```python
from build123d import *

# Parameters (mm, degrees)
CROQUIS1_R              = 1
SALIENTE_EXTRUIR1_DEPTH = 10
REDONDEO1_R             = 10


with BuildPart() as part:
    # Croquis1 → Saliente-Extruir1 (new body)
    with BuildSketch(Plane(origin=(0, 0, 0), x_dir=(1, 0, 0), z_dir=(0, 1, 0))):
        with BuildLine():
            Line((0, 100), (6.25, 95))
            Line((6.25, 95), (6.25, 10.825317547))
            ThreePointArc((6.25, 10.825317547), (10.825317547, 6.25), (12.5, 0))
            Line((12.5, 0), (12.5, 100))
            Line((12.5, 100), (0, 100))
        make_face()
        with BuildLine():
            ThreePointArc((12.5, 0), (10.825317547, 6.25), (6.25, 10.825317547))
            Line((6.25, 10.825317547), (6.25, 0))
            Line((6.25, 0), (6.5, 0))
            ThreePointArc((6.5, 0), (7.5, 1), (8.5, 0))
            Line((8.5, 0), (12.5, 0))
        make_face()
        with BuildLine():
            Line((6.25, 0), (6.25, 10.825317547))
            ThreePointArc((6.25, 10.825317547), (3.235238064, 12.074072829), (0, 12.5))
            Line((0, 12.5), (0, 8.5))
            ThreePointArc((0, 8.5), (0.707106781, 8.207106781), (1, 7.5))
            ThreePointArc((1, 7.5), (0.707106781, 6.792893219), (0, 6.5))
            Line((0, 6.5), (0, 3.75))
            ThreePointArc((0, 3.75), (2.651650429, 2.651650429), (3.75, 0))
            Line((3.75, 0), (6.25, 0))
        make_face()
        with BuildLine():
            Line((0, 8.5), (0, 12.5))
            ThreePointArc((0, 12.5), (-8.838834765, -8.838834765), (12.5, 0))
            Line((12.5, 0), (8.5, 0))
            ThreePointArc((8.5, 0), (7.5, -1), (6.5, 0))
            Line((6.5, 0), (6.25, 0))
            Line((6.25, 0), (3.75, 0))
            ThreePointArc((3.75, 0), (-2.651650429, -2.651650429), (0, 3.75))
            Line((0, 3.75), (0, 6.5))
            ThreePointArc((0, 6.5), (-1, 7.5), (0, 8.5))
        make_face()
        with Locations((-7.5, 0)):
            Circle(CROQUIS1_R, mode=Mode.SUBTRACT)
        with Locations((0, -7.5)):
            Circle(CROQUIS1_R, mode=Mode.SUBTRACT)
    extrude(amount=SALIENTE_EXTRUIR1_DEPTH)

    # Redondeo1
    redondeo1_edges = [part.edges().sort_by_distance(p)[0] for p in [
        (6.25, 5, -10.825317547),
    ]]
    fillet(redondeo1_edges, radius=REDONDEO1_R)


solid = part.part
```
The model under review builds one solid part; all positions refer to its coordinate system, in mm. A direction names the side the tool comes from. Coordinates: 2 decimals unless noted, no trailing zeros. Write each loop counter-clockwise with the first axis right and the second up, starting at its lowest first coordinate (ties: lowest second). Pieces come first, ordered by that corner, then holes.
1) Machinability: for faces 1 (the face through (6.4, 10, -31.5)), 2 (the face through (6.25, 5, -59)), which of the approach directions +Z, -Z, +X, -X, +Y, -Y give a long, thin tool a straight path to every point of the face, cutting with its end or side? Answer none if there is none.
2) We need section A-A on x = -7.5. State the section outline as (y, z) points.
3) We need section D-D on z = -80. State the section outline as (x, y) points.
4) Clearance check with flat-ended pins moving along their axes: pin 1 Ø3 at (x, z) = (7.5, 0) entering from -Y; pin 2 Ø3 at (y, z) = (3.5, -83) entering from -X; pin 3 Ø5 at (x, y) = (-10, 5.5) entering from -Z; pin 4 Ø1.8 at (x, z) = (0, 7.5) entering from +Y. State where each tip first meets the part, or that it passes through.
5) We need section B-B on z = 7.5. State the section outline as (x, y) points, then the cut area to 3 significant figures.
6) We need section C-C on y = 2. Count the separate pieces of the cut face and the enclosed holes in it, then the cut area to 3 significant figures.
7) The part is to be moulded in two halves that separate along X. For faces 3 (the face through (12.5, 5, -49)), 4 (the face through (-8.3, 4.9, 0.6)), 5 (the face through (3.081, 4.93, -97.535)), say which applies: pulls with the +X half, pulls with the -X half, needs draft (parallel to the pull), parting line crosses it, or undercut.
8) To check wall thickness, follow probe 1 along Z at (x, y) = (7.5, 8); probe 2 along Z at (x, y) = (2.5, 4.5); probe 3 along X at (y, z) = (9.75, -63). State the ranges of each line that lie inside material, in increasing order.
Answer list:
1. face 1: +Z, -Z, +X, -X, +Y
1. face 2: -X, +Y, -Y
2. outline: (0, -10) - (10, -10) - (10, -1) - (0, -1) - close; (0, 1) - (10, 1) - (10, 10) - (0, 10) - close
3. outline: (6.25, 0) - (12.5, 0) - (12.5, 10) - (6.25, 10) - close
4. pin 1: stops at y = 0
4. pin 2: stops at x = 6.25
4. pin 3: stops at z = -10
4. pin 4: passes through
5. outline: (-10, 0) - (-1, 0) - (-1, 10) - (-10, 10) - close; (1, 0) - (10, 0) - (10, 10) - (1, 10) - close
5. area: 180 mm2
6. separate pieces: 1
6. enclosed holes: 5
6. area: 1,050 mm2
7. face 3: pulls with the +X half
7. face 4: undercut
7. face 5: pulls with the -X half
8. probe 1: z = -100 to -1, 1 to 10
8. probe 2: z = -100 to -98, -14.38 to -2.8, 2.8 to 12.25
8. probe 3: x = 6.25 to 12.5
